Check sheet for the modelled part. Datum: model origin and axes. Units: mm. A direction names the side the tool comes from. Round coordinates to 2 decimals unless told otherwise and drop trailing zeros. Write each loop counter-clockwise with the first axis right and the second up, starting at its lowest first coordinate (ties: lowest second). Pieces come first, ordered by that corner, then holes. Notation, with made-up numbers: (-39.75, 83) -> (8.25, 83) arc R18 cw to (8.25, 98) -> close; hole circle Ø10 at (21.25, 56). An arc over 180 degrees is marked (long way). One line per item, written item: value. Start each with the question number.
```python
from build123d import *

# Parameters (mm, degrees)
F0_R      = 32.048134
F1_DEPTH  = 2
F2_R      = 5.685229
F3_DEPTH  = 25
F4_R      = 5.933428
F5_DEPTH  = 25
F6_R      = 5.76915
F7_DEPTH  = 25
F8_R      = 5.981832
F9_DEPTH  = 25
F11_DEPTH = 1
F12_R     = 4.686623
F13_DEPTH = 25
F14_R     = 2.480316
F14_R_2   = 2.235724
F15_DEPTH = 25
F16_R     = 2.235725
F16_R_2   = 2.235727
F17_DEPTH = 25
F18_R     = 2.235725
F18_R_2   = 2.480314
F19_DEPTH = 25
F20_R     = 2.480316
F20_R_2   = 2.235727
F21_DEPTH = 25


with BuildPart() as f1:
    # F0 (on Top) → F1 (new body)
    with BuildSketch(Plane.XY):
        Circle(F0_R)
    extrude(amount=-F1_DEPTH)

    # F2 (on face) → F3 (cut)
    with BuildSketch(Plane(origin=(0, 0, -2), x_dir=(1, 0, 0), z_dir=(0, 0, -1))):
        with Locations((0, -24.338091)):
            Circle(F2_R)
    extrude(amount=-F3_DEPTH, mode=Mode.SUBTRACT)

    # F4 (on face) → F5 (cut)
    with BuildSketch(Plane(origin=(0, 0, -2), x_dir=(1, 0, 0), z_dir=(0, 0, -1))):
        with Locations((23.407973, 0)):
            Circle(F4_R)
    extrude(amount=-F5_DEPTH, mode=Mode.SUBTRACT)

    # F6 (on face) → F7 (cut)
    with BuildSketch(Plane(origin=(0, 0, -2), x_dir=(1, 0, 0), z_dir=(0, 0, -1))):
        with Locations((0, 23.407973)):
            Circle(F6_R)
    extrude(amount=-F7_DEPTH, mode=Mode.SUBTRACT)

    # F8 (on face) → F9 (cut)
    with BuildSketch(Plane(origin=(0, 0, -2), x_dir=(1, 0, 0), z_dir=(0, 0, -1))):
        with Locations((-24.338093, 0)):
            Circle(F8_R)
    extrude(amount=-F9_DEPTH, mode=Mode.SUBTRACT)

    # F10 (on face) → F11 (join)
    with BuildSketch(Plane(origin=(0, 0, -2), x_dir=(1, 0, 0), z_dir=(0, 0, -1))):
        Polygon((-5.817543, -10.07628), (5.817543, -10.07628), (11.635086, 0), (5.817543, 10.07628), (-5.817543, 10.07628), (-11.635086, 0), align=None)
    extrude(amount=F11_DEPTH)

    # F12 (on face) → F13 (cut)
    with BuildSketch(Plane(origin=(0, 0, -3), x_dir=(1, 0, 0), z_dir=(0, 0, -1))):
        Circle(F12_R)
    extrude(amount=-F13_DEPTH, mode=Mode.SUBTRACT)

    # F14 (on face) → F15 (cut)
    with BuildSketch(Plane(origin=(0, 0, -2), x_dir=(1, 0, 0), z_dir=(0, 0, -1))):
        with Locations((-11.316436, -13.176673)):
            Circle(F14_R)
        with Locations((-17.517224, -19.377461)):
            Circle(F14_R_2)
    extrude(amount=-F15_DEPTH, mode=Mode.SUBTRACT)

    # F16 (on face) → F17 (cut)
    with BuildSketch(Plane(origin=(0, 0, -2), x_dir=(1, 0, 0), z_dir=(0, 0, -1))):
        with Locations((12.866635, -11.936517)):
            Circle(F16_R)
        with Locations((17.827265, -18.137304)):
            Circle(F16_R_2)
    extrude(amount=-F17_DEPTH, mode=Mode.SUBTRACT)

    # F18 (on face) → F19 (cut)
    with BuildSketch(Plane(origin=(0, 0, -2), x_dir=(1, 0, 0), z_dir=(0, 0, -1))):
        with Locations((11.006399, 12.866634)):
            Circle(F18_R)
        with Locations((16.587107, 20.30758)):
            Circle(F18_R_2)
    extrude(amount=-F19_DEPTH, mode=Mode.SUBTRACT)

    # F20 (on Top) → F21 (cut)
    with BuildSketch(Plane.XY):
        with Locations((-12.866635, -12.866634)):
            Circle(F20_R)
        with Locations((-16.587107, -21.547737)):
            Circle(F20_R_2)
    extrude(amount=-F21_DEPTH, mode=Mode.SUBTRACT)


solid = f1.part
```
1. Cross-section at B-B (z = -0.6). Give the number of separate pieces and of enclosed holes in the cut face, plus the area to 3 significant figures.
2. Material ranges on probe 1 along Y at (x, z) = (0, -1.15); probe 2 along X at (y, z) = (5.5, -1.3); probe 3 along X at (y, z) = (-5, -0.3), recorded low to high.
3. Release check for a two-part mould opening along Y. For faces 4 (the face through (-18.81, 2.29, -1.01)), 5 (the face through (8.767, -4.968, -2.493)), 6 (the face through (7, 0, 0)) record: +Y half, -Y half, draft (parallel to the pull), parting line (faces both ways), or undercut.
4. Access from +Z, -Z, +X, -X, +Y, -Y to the whole of each face (thin tool, end or side, straight path). Record for faces 1 (the face through (-8.686, -5.109, -2.493)), 2 (the face through (8.686, 5.109, -2.493)), 3 (the face through (-8.767, 4.968, -2.493)).
5. Depth check by flat-ended pin: pin 1 Ø1.1 at (x, z) = (-1.5, -2.5) entering from +Y; pin 2 Ø1.5 at (y, z) = (19, -1.5) entering from +X; pin 3 Ø8.5 at (x, y) = (0, 0) entering from -Z; pin 4 Ø19 at (x, y) = (-24.34, 0) entering from -Z. Enter the tip coordinate at first touch or a pass-through.
6. Cross-section at D-D (y = -1.5). Record the cut outline in (x, z), plus the area to 3 significant figures.
7. Cross-section at A-A (x = 0). Record the cut outline in (y, z), plus the area to 3 significant figures.
8. Cross-section at C-C (x = -22). Record the cut outline in (y, z), plus the area to 3 significant figures.
Working result:
1. separate pieces: 1
1. enclosed holes: 13
1. area: 2,590 mm^2
2. probe 1: y = -32.05 to -29.18, -17.64 to -4.69, 4.69 to 18.65, 30.02 to 32.05
2. probe 2: x = -31.57 to -26.69, -21.99 to 21.18, 25.63 to 31.57
2. probe 3: x = -31.66 to -27.62, -21.05 to 20.21, 26.6 to 31.66
3. face 4: undercut
3. face 5: -Y half
3. face 6: draft
4. face 1: -Z, -X, -Y
4. face 2: -Z, +X, +Y
4. face 3: -Z, -X, +Y
5. pin 1: stops at y = 32.02
5. pin 2: stops at x = 26.34
5. pin 3: passes through
5. pin 4: stops at z = -2
6. outline: (-32.01, -2) -> (-30.13, -2) -> (-30.13, 0) -> (-32.01, 0) -> close; (-18.55, -2) -> (-10.77, -2) -> (-10.77, -3) -> (-4.44, -3) -> (-4.44, 0) -> (-18.55, 0) -> close; (4.44, -3) -> (10.77, -3) -> (10.77, -2) -> (17.67, -2) -> (17.67, 0) -> (4.44, 0) -> close; (29.15, -2) -> (32.01, -2) -> (32.01, 0) -> (29.15, 0) -> close
6. area: 76.8 mm^2
7. outline: (-32.05, -2) -> (-29.18, -2) -> (-29.18, 0) -> (-32.05, 0) -> close; (-17.64, -2) -> (-10.08, -2) -> (-10.08, -3) -> (-4.69, -3) -> (-4.69, 0) -> (-17.64, 0) -> close; (4.69, -3) -> (10.08, -3) -> (10.08, -2) -> (18.65, -2) -> (18.65, 0) -> (4.69, 0) -> close; (30.02, -2) -> (32.05, -2) -> (32.05, 0) -> (30.02, 0) -> close
7. area: 74.4 mm^2
8. outline: (-23.3, -2) -> (-5.51, -2) -> (-5.51, 0) -> (-23.3, 0) -> close; (5.51, -2) -> (23.3, -2) -> (23.3, 0) -> (5.51, 0) -> close
8. area: 71.2 mm^2
